```python
from build123d import *

# Parameters (mm, degrees)
SKETCH_1_W               = 80
SKETCH_1_H               = 80
EXTRUDE_1_DEPTH          = 10
FILLET_1_R               = 10
CUT_EXTRUDE_2_DEPTH      = 58.445626465
SKETCH_4_R               = 5
CUT_EXTRUDE_5_DEPTH      = 58.445626465
SKETCH_5_R               = 1.6
CUT_EXTRUDE_3_DEPTH      = 58.445626465
SKETCH_6_W               = 10
SKETCH_6_H               = 10
EXTRUDE_3_DEPTH          = 10
CUT_EXTRUDE_4_DEPTH      = 65.807406984
CUT_EXTRUDE_4_DEPTH_BACK = 65.807406984
SKETCH_7_R               = 1.6


with BuildPart() as part:
    # ｽｹｯﾁ1 → ﾎﾞｽ - 押し出し1 (new body)
    with BuildSketch(Plane(origin=(0, 0, 0), x_dir=(1, 0, 0), z_dir=(0, 1, 0))):
        Rectangle(SKETCH_1_W, SKETCH_1_H)
    extrude(amount=EXTRUDE_1_DEPTH)

    # ﾌｨﾚｯﾄ1
    fillet_1_edges = [part.edges().sort_by_distance(p)[0] for p in [
        (40, 5, 40),
        (-40, 5, 40),
        (-40, 5, -40),
        (40, 5, -40),
    ]]
    fillet(fillet_1_edges, radius=FILLET_1_R)

    # ｽｹｯﾁ3 → ｶｯﾄ - 押し出し2 (cut, through all)
    with BuildSketch(Plane(origin=(0, 10, 0), x_dir=(1, 0, 0), z_dir=(0, 1, 0))):
        with BuildLine():
            Line((-4, -25), (4, -25))
            ThreePointArc((4, -25), (11.071067812, -22.071067812), (14, -15))
            Line((14, -15), (14, 15))
            ThreePointArc((14, 15), (11.071067812, 22.071067812), (4, 25))
            Line((4, 25), (-4, 25))
            ThreePointArc((-4, 25), (-11.071067812, 22.071067812), (-14, 15))
            Line((-14, 15), (-14, -15))
            ThreePointArc((-14, -15), (-11.071067812, -22.071067812), (-4, -25))
        make_face()
    extrude(amount=-CUT_EXTRUDE_2_DEPTH, mode=Mode.SUBTRACT)

    # ｽｹｯﾁ4 → ｶｯﾄ - 押し出し5 (cut, through all)
    with BuildSketch(Plane(origin=(0, 10, 0), x_dir=(1, 0, 0), z_dir=(0, 1, 0))):
        with Locations(Location((-30, 30, 0), (0, 0, 270))):
            Circle(SKETCH_4_R)
        with Locations(Location((30, 30, 0), (0, 0, 270))):
            Circle(SKETCH_4_R)
        with Locations(Location((-30, -30, 0), (0, 0, 270))):
            Circle(SKETCH_4_R)
        with Locations(Location((30, -30, 0), (0, 0, 270))):
            Circle(SKETCH_4_R)
    extrude(amount=-CUT_EXTRUDE_5_DEPTH, mode=Mode.SUBTRACT)

    # ｽｹｯﾁ5 → ｶｯﾄ - 押し出し3 (cut, through all)
    with BuildSketch(Plane.XZ):
        with Locations(Location((27, 14.5, 0), (0, 0, 270))):
            Circle(SKETCH_5_R)
        with Locations(Location((-27, 14.5, 0), (0, 0, 270))):
            Circle(SKETCH_5_R)
        with Locations(Location((-27, -14.5, 0), (0, 0, 270))):
            Circle(SKETCH_5_R)
        with Locations(Location((27, -14.5, 0), (0, 0, 270))):
            Circle(SKETCH_5_R)
    extrude(amount=-CUT_EXTRUDE_3_DEPTH, mode=Mode.SUBTRACT)

    # ｽｹｯﾁ6 → ﾎﾞｽ - 押し出し3 (add)
    with BuildSketch(Plane(origin=(0, 0, -40), x_dir=(-1, 0, 0), z_dir=(0, 0, -1))):
        with Locations((-15, 5)):
            Rectangle(SKETCH_6_W, SKETCH_6_H)
        with Locations((15, 5)):
            Rectangle(SKETCH_6_W, SKETCH_6_H)
    extrude(amount=EXTRUDE_3_DEPTH)

    # ｽｹｯﾁ7 → ｶｯﾄ - 押し出し4 (cut, two sides: drawn at the far end of the back side and taken through both)
    with BuildSketch(Plane(origin=(0, 0, 0), x_dir=(0, 0, -1), z_dir=(1, 0, 0)).offset(-CUT_EXTRUDE_4_DEPTH_BACK)):
        with Locations((45, 5)):
            Circle(SKETCH_7_R)
    extrude(amount=CUT_EXTRUDE_4_DEPTH + CUT_EXTRUDE_4_DEPTH_BACK, mode=Mode.SUBTRACT)


solid = part.part
```
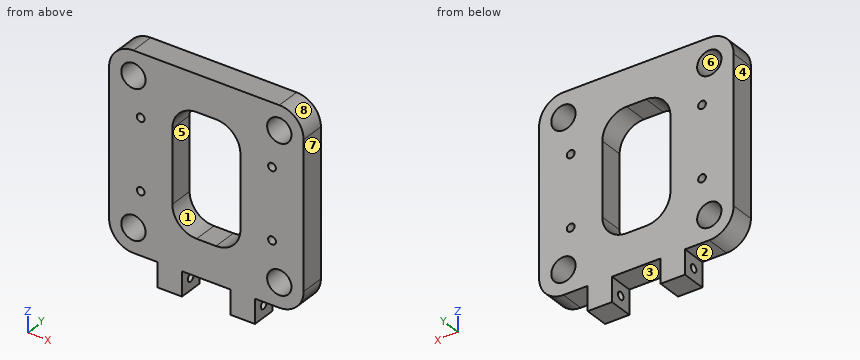
Input: part model. Units: mm. Frame: model coordinates. Face numbers are marked on the shaded views. A direction names the side the tool comes from. Round coordinates to 2 decimals unless told otherwise and drop trailing zeros. Loops run counter-clockwise (first coordinate to the right, second up) from the corner with the lowest first, then second, coordinate; pieces in that order, holes last. Notation, with made-up numbers: (36, 78) - (84, 78) arc R19 cw to (84, 104) - close; hole circle Ø6 at (88, 55.5). An arc over 180 degrees is marked (long way). One line per item, written item: value. Start each with the question number.
(1) Section C-C, the plane x = -7.5. Return loops of the section in (y, z), plus the area to 3 significant figures.
(2) Section A-A, the plane x = 27. Return loops of the section in (y, z).
(3) Ray query, line 1 (X direction, y = 2.5, z = -30); line 2 (X direction, y = 7.25, z = 5.5); line 3 (Z direction, x = 3, y = 5.75). Return the intervals inside material, ascending. Write a range as [from, to].
(4) Contact query for flat-ended pins moving along their axis: P1, Ø3.5, axis at y = 5, z = -45, coming from the +X side; P2, Ø5, axis at y = 2.5, z = -47.5, coming from the -X side. Output: stop coordinate, or through.
(5) Access query for the marked faces 1, 2, 3 and 4. Directions: +Z, -Z, +X, -X, +Y, -Y. A direction counts if a zero-diameter tool reaches every point of the face in a straight line with its end or side. Return the directions, or none.
(6) Draft query along Z for the marked faces 5, 6, 7 and 8. Return one class per face: +Z half, -Z half, draft (parallel to the pull), parting line (faces both ways), or undercut.
(7) Section B-B, the plane z = -0.5. Return loops of the section in (x, y), plus the area to 3 significant figures.
(8) Section D-D, the plane z = -36.5. Return loops of the section in (x, y).
Results below:
1. outline: (0, -40) - (10, -40) - (10, -24.37) - (0, -24.37) - close; (0, 24.37) - (10, 24.37) - (10, 40) - (0, 40) - close
1. area: 313 mm^2
2. outline: (0, -40) - (10, -40) - (10, -34) - (0, -34) - close; (0, -26) - (10, -26) - (10, -16.1) - (0, -16.1) - close; (0, -12.9) - (10, -12.9) - (10, 12.9) - (0, 12.9) - close; (0, 16.1) - (10, 16.1) - (10, 26) - (0, 26) - close; (0, 34) - (10, 34) - (10, 40) - (0, 40) - close
3. line 1: [-40, -35], [-25, 25], [35, 40]
3. line 2: [-40, -14], [14, 40]
3. line 3: [-40, -25], [25, 40]
4. P1: x = 20
4. P2: x = -20
5. face 1: +Y, -Y
5. face 2: -Z, -X, +Y, -Y
5. face 3: -Z, +Y, -Y
5. face 4: +Z, -Z, -X, +Y, -Y
6. face 5: undercut
6. face 6: undercut
6. face 7: draft
6. face 8: +Z half
7. outline: (-40, 0) - (-14, 0) - (-14, 10) - (-40, 10) - close; (14, 0) - (40, 0) - (40, 10) - (14, 10) - close
7. area: 520 mm^2
8. outline: (-37.6, 0) - (37.6, 0) - (37.6, 10) - (-37.6, 10) - close
